Verification items for the finished model (mm, model axes). A direction names the side the tool comes from. Coordinates: 2 decimals unless noted, no trailing zeros. Order: outer loops, then holes, each group sorted by start corner. A loop starts at its lowest first (then second) coordinate and runs counter-clockwise, first axis right, second up. Notation, with made-up numbers: (88.25, 84) -> (143.25, 84) arc R21 ccw to (143.25, 109) -> close; hole circle Ø9 at (39, 24). An arc over 180 degrees is marked (long way). Write item = value, one per line. Start each with the question number.
1. Go/stop test with flat-tipped pins: P1, Ø8.5, axis at y = -25, z = 8, coming from the +X side; P2, Ø3, axis at x = 17.5, z = 15.5, coming from the -Y side; P3, Ø5, axis at y = -8.26, z = 11.84, coming from the -X side; P4, Ø14.5, axis at y = -2.6, z = 17.5, coming from the +X side. Record where each tip stops, or that it passes through.
2. Cross-section at D-D on z = 8. Record the cut outline in (x, y).
3. Thickness scan on line 1 along X through (y, z) = (-18.5, 33); line 2 along Y through (x, z) = (13.5, 11); line 3 along Y through (x, z) = (-11.5, 17.5). Record the ranges inside material, lowest first. Write a range as from..to.
4. Cross-section at C-C on z = 16. Record the cut outline in (x, y), plus the area to 3 significant figures.
5. Set-up check for faces 1 (the cylindrical face through (1.68, -9.72, 22.83)), 2 (the flat face through (-25, -15, 17)), 3 (the cylindrical face through (-14.584, -2.371, 12.305)), 4 (the flat face through (-10.1, -25, 17)): record each of +Z, -Z, +X, -X, +Y, -Y from which the full face is reachable in a straight line by a thin tool's end or side.
6. Cross-section at B-B on x = -23. Record the cut outline in (y, z), plus the area to 3 significant figures.
7. Release check for a two-part mould opening along Z. For faces 5 (the cylindrical face through (8.2, -5.3, 21.1)), 6 (the flat face through (-5, -5, 35)), 7 (the flat face through (0, -15, 17)) record: +Z half, -Z half, draft (parallel to the pull), parting line (faces both ways), or undercut.
8. Cross-section at A-A on y = -19. Record the cut outline in (x, z).
from build123d import *

# Parameters (mm, degrees)
EXTRUDE_1_DEPTH     = 35
HOLE_WIZARD_1_D     = 9
SKETCH_12_R         = 1.5
CUT_EXTRUDE_1_DEPTH = 70.548831766
SKETCH_15_R         = 5.2
CUT_EXTRUDE_4_DEPTH = 16
SKETCH_14_R         = 11.75
CUT_EXTRUDE_3_DEPTH = 4
HOLE_WIZARD_2_D     = 5.2
HOLE_WIZARD_2_DEPTH = 100
EXTRUDE_START       = 10
SKETCH_18_W         = 35
SKETCH_18_H         = 30
SKETCH_18_R         = 11.75
EXTRUDE_2_DEPTH     = 10


with BuildPart() as part:
    # 草图1 → 凸台-拉伸1 (new body)
    with BuildSketch(Plane.XY):
        Polygon((15.1, -15), (15.1, -34.8), (10.1, -34.8), (10.1, -15), (-10.1, -15), (-10.1, -34.8), (-15.1, -34.8), (-15.1, -15), (-24.5, -15), (-24.5, 15), (24.5, 15), (24.5, -15), align=None)
    extrude(amount=EXTRUDE_1_DEPTH)

    # 孔1 (through all)
    with Locations(Plane.ZY.offset(24.5)):
        with Locations((17.5, -2.6)):
            Hole(HOLE_WIZARD_1_D / 2)

    # 草图12 → 切除-拉伸1 (cut, through all)
    with BuildSketch(Plane.ZY.offset(24.5)):
        with Locations((11.843145751, 3.056854249)):
            Circle(SKETCH_12_R)
        with Locations((23.156854249, 3.056854249)):
            Circle(SKETCH_12_R)
        with Locations((23.156854249, -8.256854249)):
            Circle(SKETCH_12_R)
        with Locations((11.843145751, -8.256854249)):
            Circle(SKETCH_12_R)
    extrude(amount=-CUT_EXTRUDE_1_DEPTH, mode=Mode.SUBTRACT)

    # 草图15 → 切除-拉伸4 (cut)
    with BuildSketch(Plane.ZY.offset(24.5)):
        with Locations((17.5, -2.6)):
            Circle(SKETCH_15_R)
    extrude(amount=-CUT_EXTRUDE_4_DEPTH, mode=Mode.SUBTRACT)

    # 草图14 → 切除-拉伸3 (cut)
    with BuildSketch(Plane.ZY.offset(24.5)):
        with Locations((17.5, -2.6)):
            Circle(SKETCH_14_R)
    extrude(amount=-CUT_EXTRUDE_3_DEPTH, mode=Mode.SUBTRACT)

    # 孔2
    with Locations(Plane.ZY.offset(15.1)):
        with Locations((8, -25), (27, -25)):
            Hole(HOLE_WIZARD_2_D / 2, depth=HOLE_WIZARD_2_DEPTH)

    # 草图18 → 凸台-拉伸2 (add)
    with BuildSketch(Plane.ZY.offset(24.5).offset(EXTRUDE_START)):
        with Locations((17.5, 0)):
            Rectangle(SKETCH_18_W, SKETCH_18_H)
        with Locations((17.5, -2.6)):
            Circle(SKETCH_18_R, mode=Mode.SUBTRACT)
    extrude(amount=-EXTRUDE_2_DEPTH)


solid = part.part
Worked out:
q1.P1 = 15.1
q1.P2 = -15
q1.P3 = -20.5
q1.P4 = 24.5
q2.outline = (-34.5, -15) -> (-15.1, -15) -> (-15.1, -22.4) -> (-10.1, -22.4) -> (-10.1, -15) -> (10.1, -15) -> (10.1, -22.4) -> (15.1, -22.4) -> (15.1, -15) -> (24.5, -15) -> (24.5, 15) -> (-34.5, 15) -> (-34.5, 4.31) -> (-20.5, 4.31) -> (-20.5, -9.51) -> (-34.5, -9.51) -> close; (-15.1, -34.8) -> (-10.1, -34.8) -> (-10.1, -27.6) -> (-15.1, -27.6) -> close; (10.1, -34.8) -> (15.1, -34.8) -> (15.1, -27.6) -> (10.1, -27.6) -> close
q3.line_1 = -15.1..-10.1, 10.1..15.1
q3.line_2 = -34.8..-9.5, -7.02..1.82, 4.3..15
q3.line_3 = -34.8..-7.8, 2.6..15
q4.outline = (-34.5, -15) -> (-15.1, -15) -> (-15.1, -34.8) -> (-10.1, -34.8) -> (-10.1, -15) -> (10.1, -15) -> (10.1, -34.8) -> (15.1, -34.8) -> (15.1, -15) -> (24.5, -15) -> (24.5, -6.84) -> (-8.5, -6.84) -> (-8.5, -7.58) -> (-20.5, -7.58) -> (-20.5, -14.25) -> (-34.5, -14.25) -> close; (-34.5, 9.05) -> (-20.5, 9.05) -> (-20.5, 2.38) -> (-8.5, 2.38) -> (-8.5, 1.64) -> (24.5, 1.64) -> (24.5, 15) -> (-34.5, 15) -> close
q4.area = 1,240 mm²
q5.face_1 = +X, -X
q5.face_2 = +Z, -Z, -X, -Y
q5.face_3 = -X
q5.face_4 = +Z, -Z, -Y
q6.outline = (-15, 0) -> (15, 0) -> (15, 35) -> (-15, 35) -> close; hole circle Ø23.5 at (-2.6, 17.5)
q6.area = 616 mm²
q7.face_5 = undercut
q7.face_6 = +Z half
q7.face_7 = draft
q8.outline = (-15.1, 0) -> (-10.1, 0) -> (-10.1, 35) -> (-15.1, 35) -> close; (10.1, 0) -> (15.1, 0) -> (15.1, 35) -> (10.1, 35) -> close
